Design review of the part built by this model. Coordinates are the model's own, in mm. A direction names the side the tool comes from. Give positions to 0.01 mm unless a question says otherwise; leave off trailing zeros. Order: outer loops, then holes, each group sorted by start corner. A loop starts at its lowest first (then second) coordinate and runs counter-clockwise, first axis right, second up. Notation, with made-up numbers: (26.25, 54.5) -> (55.25, 54.5) arc R21 cw to (55.25, 71.5) -> close; hole circle Ø5 at (72, 17). An arc over 180 degrees is marked (long way). One line per item, written item: value. Start each with the question number.
1) Consider section A-A (y = 27.5). State the section outline as (x, z) points.
2) Consider section D-D (x = 1.25). State the section outline as (y, z) points.
3) Consider section C-C (z = -26). State the section outline as (x, y) points, plus the area to 3 significant figures.
4) Consider section B-B (x = 5.75). State the section outline as (y, z) points.
5) Wall thickness on line 1 along Y through (x, z) = (1.6, -26.6); line 2 along X through (y, z) = (42.5, -21); line 3 along Y through (x, z) = (1.5, -32.5): over which ranges is each line inside the solid? List them lowest first. Write a range as from..to.
6) For pin 1 (2 mm diameter, centred on x = 1.5, z = -33, fed in from +Y); pin 2 (2 mm diameter, centred on x = 1, z = -36.5, fed in from -Y); pin 3 (2 mm diameter, centred on x = 3, y = 26.5, fed in from +Z); pin 4 (0.5 mm diameter, centred on x = 3.5, y = 7, fed in from +Z), all flat-tipped, find the tip position at first contact; note any pin that passes through.
7) The part is to be moulded in two halves that separate along Y. For faces 1 (the face through (1, 14.5, -33)), 2 (the face through (5, 14.5, -24)), 3 (the face through (5, 40.5, -24)), 4 (the face through (3, 48, -27.1)), say which applies: released by +Y, released by -Y, zero draft, split by the parting line, or undercut.
8) Tool access review of faces 5 (the face through (6, 7, -18.8)), 6 (the face through (1, 40.5, -33)), 7 (the face through (3, 48, -24.6)), 8 (the face through (3, 7, -27.1)): name each direction out of +Z, -Z, +X, -X, +Y, -Y from which nothing blocks a thin tool from reaching the whole face with its end or side.
Autodesk Inventor part; units mm, degrees
ref_plane "YZ Plane" through (0, 0, 0) normal (1, 0, 0) x (0, 1, 0)
ref_plane "XZ Plane" through (0, 0, 0) normal (0, 1, 0) x (-1, 0, 0)
ref_plane "XY Plane" through (0, 0, 0) normal (0, 0, 1) x (1, 0, 0)
sketch "Sketch1" plane through (0, 0, 0) normal (0, 1, 0) x (-1, 0, 0)
  line L0 (0, 27.1) -> (0, -27.1)
  line L1 (0, 27.1) -> (-6.8, 27.1)
  line L2 (-6.8, 27.1) -> (-6.8, 18.8)
  line L3 (-6.8, 18.8) -> (-4.3, 18.8)
  line L4 (-4.3, 18.8) -> (-4.3, 24.6)
  line L5 (-4.3, 24.6) -> (-2.5, 24.6)
  line L6 (-2.5, 24.6) -> (-2.5, 0)
  line L7 (0, -27.1) -> (-6.8, -27.1)
  line L8 (-6.8, -27.1) -> (-6.8, -18.8)
  line L9 (-6.8, -18.8) -> (-4.3, -18.8)
  line L10 (-4.3, -18.8) -> (-4.3, -24.6)
  line L11 (-4.3, -24.6) -> (-2.5, -24.6)
  line L12 (-2.5, -24.6) -> (-2.5, 0)
  point P0 (0, 0)
  dimension "d0" = 54.2
  dimension "d1" = 6.8
  dimension "d2" = 8.3
  dimension "d3" = 2.5
  dimension "d4" = 5.8
  dimension "d5" = 1.8
  dimension "d6" = 8.3
  dimension "d7" = 5.8
extrude "Extrusion1" add sketch "Sketch1" along normal blind 14.5
sketch "Sketch2" plane through (0, 14.5, 0) normal (0, 1, 0) x (1, 0, 0)
  line L0 (2.5, -24.6) -> (2.5, 24.6)
  line L1 (2.5, 0) -> (2.5, 39.5)
  line L2 (2.5, 39.5) -> (0, 39.5)
  line L3 (0, 39.5) -> (0, 0)
  line L4 (0, 0) -> (0, -39.5)
  line L5 (0, 27.1) -> (0, -27.1)
  line L6 (0, -39.5) -> (2.5, -39.5)
  line L7 (2.5, -39.5) -> (2.5, 0)
  dimension "d10" = 39.5
  dimension "d11" = 39.5
extrude "Extrusion2" add sketch "Sketch2" along normal blind 26
sketch "Sketch3" plane through (0, 40.5, 0) normal (0, 1, 0) x (1, 0, 0)
  line L0 (2.5, -24.6) -> (2.5, 24.6)
  line L1 (2.5, 0) -> (2.5, 24.6558)
  line L2 (0, 27.1) -> (0, -27.1)
  line L3 (4.3, -24.6) -> (2.5, -24.6)
  line L4 (6.8, -18.8) -> (4.3, -18.8)
  line L5 (4.3, -24.6) -> (4.3, -18.8)
  line L6 (4.3, -18.8) -> (6.8, -18.8)
  line L7 (6.8, -18.8) -> (6.8, -27.1)
  line L8 (6.8, -27.1) -> (2.5, -27.1)
  line L9 (2.5, 0) -> (2.5, 24.6558)
  line L10 (2.5, 24.6) -> (4.3, 24.6)
  line L11 (4.3, 18.8) -> (6.8, 18.8)
  line L12 (4.3, 24.6) -> (4.3, 18.8)
  line L13 (4.3, 18.8) -> (6.8, 18.8)
  line L14 (6.8, 18.8) -> (6.8, 27.1)
  line L15 (6.8, 27.1) -> (0, 27.1)
  line L16 (0, 27.1) -> (0, -27.1)
  line L17 (6.8, -27.1) -> (0, -27.1)
  line L18 (4.3, -24.6) -> (2.5, -24.6)
  point P0 (0, 0)
extrude "Extrusion3" add sketch "Sketch3" along normal blind 14.5
sketch "Sketch4" plane through (2.5, 0, 24.6) normal (1, 0, 0) x (0, 0, -1)
  line L0 (64.1, 14.5) -> (64.1, 40.5)
  line L1 (-14.9, 14.5) -> (-14.9, 40.5)
  line L2 (-14.9, 27.5) -> (-1.5, 27.5)
  circle A0 centre (-1.5, 27.5) radius 1.5
  line L3 (64.1, 14.5) -> (64.1, 40.5)
  line L4 (64.1, 27.5) -> (51.2, 27.5)
  circle A1 centre (51.2, 27.5) radius 1.5
  point P0 (24.6, 0)
  dimension "d18" = 13.4
  dimension "d19" = 3
  dimension "d31" = 12.9
extrude "Extrusion4" cut sketch "Sketch4" against normal blind 4.5
sketch "Sketch5" plane through (0, 0, -27.1) normal (-1, 0, 0) x (0, 0, 1)
  line L0 (27.1, 0) -> (21.3, 0)
  line L1 (51.7, 0) -> (2.5, 0)
  line L2 (21.3, 0) -> (21.3, 55)
  line L3 (51.7, 55) -> (2.5, 55)
  line L4 (27.1, 55) -> (32.9, 55)
  line L5 (32.9, 55) -> (32.9, 0)
  line L6 (32.9, 0) -> (27.1, 0)
  dimension "d22" = 5.8
  dimension "d23" = 5.8
extrude "Extrusion5" cut sketch "Sketch5" against normal blind 62.3875
sketch "Sketch6" plane through (0, 0, 5.8) normal (0, 0, -1) x (-1, 0, 0)
  point P0 (0, 0)
sketch "Sketch7" plane through (0, 14.5, 27.1) normal (-1, 0, 0) x (0, 0, 1)
  line L0 (-21.3, -14.5) -> (0, -14.5)
  line L1 (-21.3, -14.5) -> (18.5957, -14.5)
  line L2 (18.5957, -14.5) -> (18.5957, 49.9868)
  line L3 (18.5957, 49.9868) -> (-21.3, 49.9868)
  line L4 (-21.3, 49.9868) -> (-21.3, -14.5)
  point P0 (-27.1, -14.5)
extrude "Extrusion6" cut sketch "Sketch7" against normal blind 62.3875
sketch "Sketch8" plane through (0, 0, -5.8) normal (0, 0, 1) x (1, 0, 0)
  line L0 (0, 55) -> (2.5, 55)
  line L1 (2.5, 0) -> (0, 0)
  line L2 (2.5, 55) -> (2.5, 0)
  line L3 (2.5, 0) -> (0, 0)
  line L4 (0, 0) -> (0, 55)
extrude "Extrusion7" add sketch "Sketch8" along normal blind 0.5
properties part number "cam_holder3"
Checked values:
1. outline: (0, -39.5) -> (2.5, -39.5) -> (2.5, -28.1) -> (0, -28.1) -> close; (0, -25.1) -> (2.5, -25.1) -> (2.5, -5.3) -> (0, -5.3) -> close
2. outline: (0, -27.1) -> (14.5, -27.1) -> (14.5, -39.5) -> (40.5, -39.5) -> (40.5, -27.1) -> (55, -27.1) -> (55, -5.3) -> (0, -5.3) -> close; hole circle Ø3 at (27.5, -26.6)
3. outline: (0, 0) -> (6.8, 0) -> (6.8, 14.5) -> (2.5, 14.5) -> (2.5, 26.13) -> (0, 26.13) -> close; (0, 28.87) -> (2.5, 28.87) -> (2.5, 40.5) -> (6.8, 40.5) -> (6.8, 55) -> (0, 55) -> close
3. area: 255 mm^2
4. outline: (0, -27.1) -> (14.5, -27.1) -> (14.5, -18.8) -> (0, -18.8) -> close; (40.5, -27.1) -> (55, -27.1) -> (55, -18.8) -> (40.5, -18.8) -> close
5. line 1: y = 0..26, 29..55
5. line 2: x = 0..2.5, 4.3..6.8
5. line 3: y = 14.5..40.5
6. pin 1: stops at y = 40.5
6. pin 2: stops at y = 14.5
6. pin 3: stops at z = -5.3
6. pin 4: stops at z = -24.6
7. face 1: released by -Y
7. face 2: undercut
7. face 3: undercut
7. face 4: zero draft
8. face 5: +Z, +X, +Y, -Y
8. face 6: -Z, +X, -X, +Y
8. face 7: +Z, +Y, -Y
8. face 8: -Z, +X, -X, -Y
